Part print with two shaded views. Sizes in mm from the minimum x, y, z corner. Give positions to 0.01 mm unless a question says otherwise; leave off trailing zeros. Order: outer loops, then holes, each group sorted by start corner. A loop starts at its lowest first (then second) coordinate and runs counter-clockwise, first axis right, second up. Notation, with made-up numbers: M 82,-31 L 135,-31 A23 ccw 135,5 Z; hole C -21.5,22.25 d3. An arc over 180 degrees is marked long. Return JSON: item names as keys, results as strings.
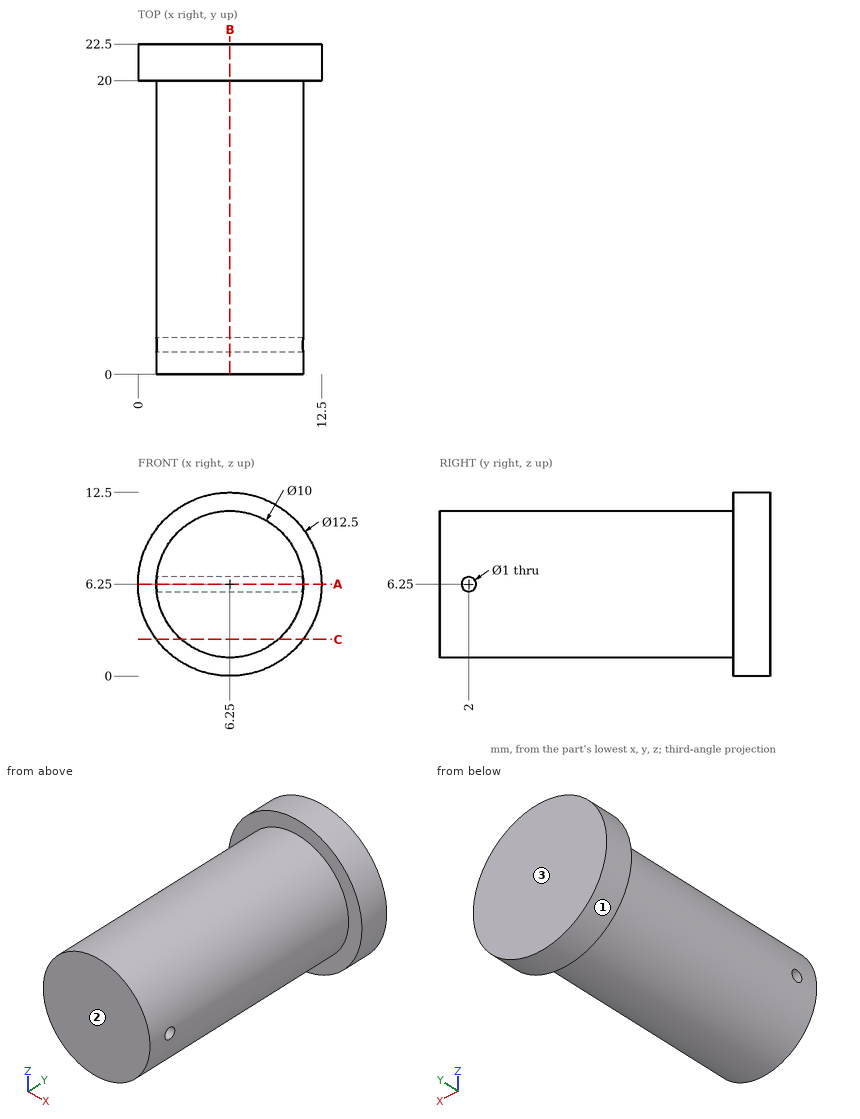
Q1. Band-saw the part on B-B (x = 6.25). Give the cut face in (y, z), then the cut area to 3 significant figures.
Established:
{"outline": "M 0,1.25 L 20,1.25 L 20,0 L 22.5,0 L 22.5,12.5 L 20,12.5 L 20,11.25 L 0,11.25 Z; hole C 2,6.25 d1", "area": "230 mm²"}
Q2. Band-saw the part on C-C (z = 2.5). Give the cut face in (x, y), then the cut area to 3 significant figures.
Established:
{"outline": "M 1.25,20 L 2.94,20 L 2.94,0 L 9.56,0 L 9.56,20 L 11.25,20 L 11.25,22.5 L 1.25,22.5 Z", "area": "157 mm²"}
Q3. Probe line 1 along Y through (x, z) = (4.5, 6.25); line 2 along Y through (x, z) = (1.5, 3); line 3 along X through (y, z) = (11.25, 6). List the from-to ranges inside material, lowest first.
Established:
{"line 1": "y = 0 to 1.5, 2.5 to 22.5", "line 2": "y = 20 to 22.5", "line 3": "x = 1.26 to 11.24"}
Q4. Band-saw the part on A-A (z = 6.25). Give the cut face in (x, y).
Established:
{"outline": "M 0,20 L 1.25,20 L 1.25,2.5 L 11.25,2.5 L 11.25,20 L 12.5,20 L 12.5,22.5 L 0,22.5 Z; M 1.25,0 L 11.25,0 L 11.25,1.5 L 1.25,1.5 Z"}
Q5. Two-plate mould, pull along Y, no slides. Class the marked faces 1, 2 and 3: +Y half, -Y half, draft (parallel to the pull), parting line (faces both ways), or undercut.
Established:
{"face 1": "draft", "face 2": "-Y half", "face 3": "+Y half"}
Q6. Pin check, flat tips, straight feed: pin 1 (3 mm diameter, centred on y = 6, z = 2, fed in from +X); pin 2 (2 mm diameter, centred on y = 3.5, z = 6, fed in from -X); pin 3 (4 mm diameter, centred on y = 16.5, z = 2.5, fed in from +X). Stop position of each tip, or through.
Established:
{"pin 1": "stops at x = 10.43", "pin 2": "stops at x = 1.25", "pin 3": "stops at x = 10.93"}
